from build123d import *

# Parameters (mm, degrees)
SKETCH1_R           = 7.5
BOSS_EXTRUDE1_DEPTH = 1070
SKETCH_1_R          = 6
EXTRUDE_1_DEPTH     = 18
SKETCH_2_R          = 4.5
EXTRUDE_2_DEPTH     = 12


with BuildPart() as part:
    # Sketch1 → Boss-Extrude1 (new body)
    with BuildSketch(Plane(origin=(0, 0, 0), x_dir=(1, 0, 0), z_dir=(0, 1, 0))):
        Circle(SKETCH1_R)
    extrude(amount=BOSS_EXTRUDE1_DEPTH)

    # Эскиз1 → Бобышка-Вытянуть1 (add)
    with BuildSketch(Plane.XZ):
        Circle(SKETCH_1_R)
    extrude(amount=EXTRUDE_1_DEPTH)

    # Эскиз2 → Бобышка-Вытянуть2 (add)
    with BuildSketch(Plane.XZ.offset(18)):
        Circle(SKETCH_2_R)
    extrude(amount=EXTRUDE_2_DEPTH)


solid = part.part
CAD build for the part. Positions are in the model's coordinates, mm. Give positions to 0.01 mm unless a question says otherwise; leave off trailing zeros. Loops run counter-clockwise (first coordinate to the right, second up) from the corner with the lowest first, then second, coordinate; pieces in that order, holes last. Notation, with made-up numbers: M -32.75,15.25 L -5.75,15.25 A24 cw -5.75,32.25 Z; hole C 33,68 d3. An arc over 180 degrees is marked long. One line per question, with ' | ' between items. Start each with the question number.
1. Saw through at A-A on y = 799.5. Give the cut face in (x, z).
2. Flat gauge pins, fed straight in: pin 1 (1 mm diameter, centred on y = 672.5, z = 4, fed in from +X); pin 2 (1.5 mm diameter, centred on x = -5, y = 262, fed in from -Z); pin 3 (1.5 mm diameter, centred on x = -6, z = -3.5, fed in from -Y). Where does each tip first touch, or does it go through?
3. Probe L1, parallel to Y at x = 4.25, z = 3.5; L2, parallel to Z at x = -0.5, y = 147; L3, parallel to Z at x = -6, y = 552. List the from-to ranges inside material, lowest first. Write a range as from..to.
4. Saw through at B-B on x = 1.25. Give the cut face in (y, z).
Result sheet:
1) outline: C 0,0 d15
2) pin 1: stops at x = 6.63 | pin 2: stops at z = -6.18 | pin 3: stops at y = 0
3) L1: y = -18..1070 | L2: z = -7.48..7.48 | L3: z = -4.5..4.5
4) outline: M -30,-4.32 L -18,-4.32 L -18,-5.87 L 0,-5.87 L 0,-7.4 L 1070,-7.4 L 1070,7.4 L 0,7.4 L 0,5.87 L -18,5.87 L -18,4.32 L -30,4.32 Z
